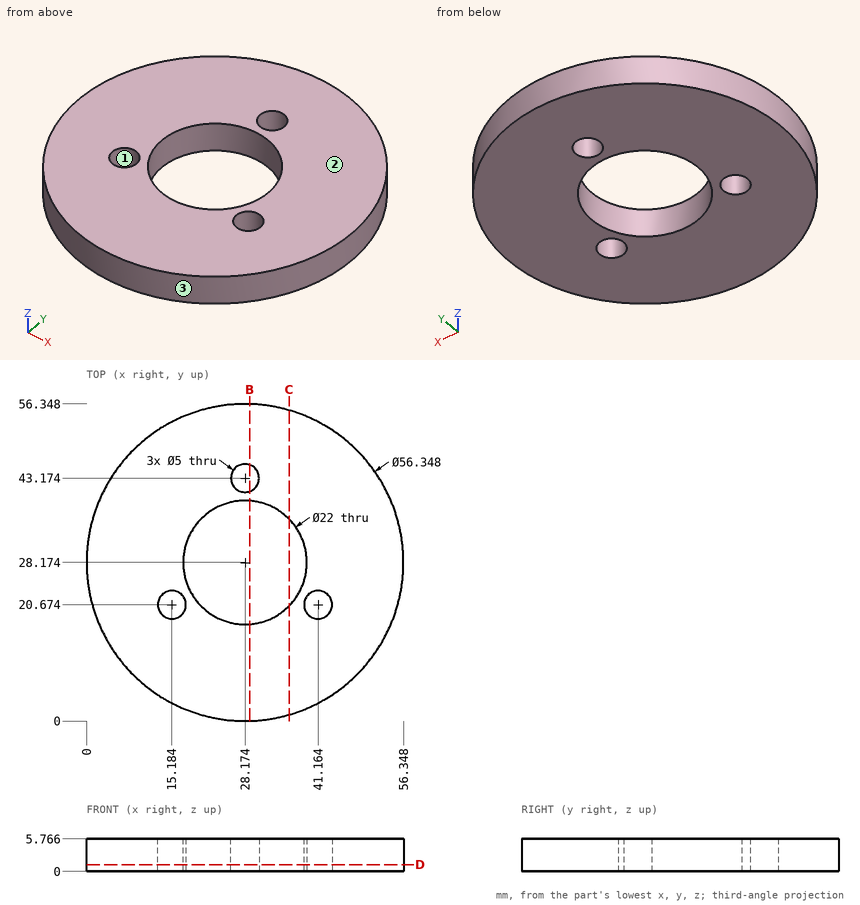
Geometry: see drawing. Coordinates: mm, zero at the bounding-box minimum. Give positions to 0.01 mm unless a question says otherwise; leave off trailing zeros. Loops run counter-clockwise (first coordinate to the right, second up) from the corner with the lowest first, then second, coordinate; pieces in that order, holes last. Notation, with made-up numbers: (46, -37) - (61, -37) arc R21 cw to (61, -5) - close; hole circle Ø10 at (40, 43.25). An arc over 180 degrees is marked (long way). Use CSV: the item, a comma, the result in double quotes. Start each with the question number.
Item 1: Line query: line 1 (X direction, y = 28.5, z = 2.2) (1 decimal); line 2 (Y direction, x = 20, z = 1.5) (1 decimal); line 3 (Y direction, x = 30, z = 3.95) (1 decimal). Output: solid intervals per line, ascending.
Item 2: Mould query, pull axis Y, two halves, no side actions, for the marked faces 1, 2 and 3. Classes: pulls with the +Y half, pulls with the -Y half, needs draft (parallel to the pull), parting line crosses it, or undercut.
Item 3: Section B-B on x = 29. Return loops of the section in (y, z) (1 decimal).
Item 4: Section D-D on z = 1.2. Return loops of the section in (x, y) (1 decimal).
Item 5: Section C-C on x = 36. Return loops of the section in (y, z) (1 decimal), then the cut area to 3 significant figures.
Item 6: Contact query for flat-ended pins moving along their axis: P1, Ø3, axis at y = 47, z = 3.5, coming from the +X side; P2, Ø3, axis at y = 39.5, z = 2, coming from the -X side; P3, Ø4.5, axis at x = 41.16, y = 20.67, coming from the -Z side. Output: stop coordinate, or through.
Ans:
1,line 1,"x = 0 to 17.2, 39.2 to 56.3"
1,line 2,"y = 1.2 to 20.8, 35.5 to 55.1"
1,line 3,"y = 0.1 to 17.3, 39 to 41.5, 44.9 to 56.3"
2,face 1,"undercut"
2,face 2,"needs draft"
2,face 3,"parting line crosses it"
3,outline,"(0, 0) - (17.2, 0) - (17.2, 5.8) - (0, 5.8) - close; (39.1, 0) - (40.8, 0) - (40.8, 5.8) - (39.1, 5.8) - close; (45.5, 0) - (56.3, 0) - (56.3, 5.8) - (45.5, 5.8) - close"
4,outline,"circle Ø56.3 at (28.2, 28.2); hole circle Ø5 at (15.2, 20.7); hole circle Ø22 at (28.2, 28.2); hole circle Ø5 at (28.2, 43.2); hole circle Ø5 at (41.2, 20.7)"
5,outline,"(1.1, 0) - (20.4, 0) - (20.4, 5.8) - (1.1, 5.8) - close; (35.9, 0) - (55.2, 0) - (55.2, 5.8) - (35.9, 5.8) - close"
5,area,"223 mm2"
6,P1,"stops at x = 50.39"
6,P2,"stops at x = 1.77"
6,P3,"passes through"
